Can you work these out from the model? Positions are in its coordinate system, mm. A direction names the side the tool comes from. Give positions to 0.01 mm unless a question says otherwise; leave off trailing zeros. Order: outer loops, then holes, each group sorted by start corner. A loop starts at its lowest first (then second) coordinate and runs counter-clockwise, first axis right, second up. Notation, with made-up numbers: M -31.5,53 L -7.5,53 A23 ccw -7.5,91 Z; hole C 15.5,0 d11. An arc over 180 degrees is marked long. One line per question, with ' | ' between items. Start each with the question number.
1) Thinking about a two-plate mould opening in X: for faces 6 (the flat face through (-5.83, 4.93, -73.97)), 7 (the flat face through (1.75, 5, 7)), 8 (the flat face through (-19.32, 4.96, -84.28)), which applies, +X half, -X half, draft (parallel to the pull), parting line (faces both ways), or undercut?
2) If we section it at A-A, the plane y = 3.25: Please give me the cut outline in (x, z), plus the area to 3 significant figures.
3) Please list where these lines run through material, in increasing order: line 1 along X through (y, z) = (2.25, -53.5); line 2 along X through (y, z) = (2.25, 7.5); line 3 along X through (y, z) = (5, -78). Write a range as [from, to].
4) If we section it at D-D, the plane x = -25.5: Please give me the cut outline in (y, z), plus the area to 3 significant figures.
5) If we section it at B-B, the plane x = -17: Please give me the cut outline in (y, z), plus the area to 3 significant figures.
6) If we section it at C-C, the plane z = 2: Please give me the cut outline in (x, y), plus the area to 4 significant figures.
7) For faces 1 (the flat face through (8.25, 5, 7)), 2 (the flat face through (-23.21, 5.04, -80.39)), 3 (the flat face through (0, 5, -27)), 4 (the flat face through (5, 1.75, 7)), 5 (the flat face through (5, 8.25, 7)), which set-ups out of +Z, -Z, +X, -X, +Y, -Y let a thin tool reach every point of the face, with its end or its side?
8) I'm going to push flat-ended pins straight in: pin 1 Ø3 at (x, z) = (4, 9) entering from +Y; pin 2 Ø1.5 at (x, y) = (0.5, 2) entering from -Z; pin 3 Ø7 at (x, z) = (4.5, 8) entering from -Y. Where does each tip first touch, or does it pass through?
Autodesk Inventor part; units mm, degrees
ref_plane "YZ Plane" through (0, 0, 0) normal (1, 0, 0) x (0, 1, 0)
ref_plane "XZ Plane" through (0, 0, 0) normal (0, 1, 0) x (-1, 0, 0)
ref_plane "XY Plane" through (0, 0, 0) normal (0, 0, 1) x (1, 0, 0)
sketch "Sketch1" plane through (0, 0, 0) normal (0, 1, 0) x (-1, 0, 0)
  line L0 (0, 0) -> (-10, 0)
  line L1 (-10, 0) -> (-10, -54)
  line L2 (0, -54) -> (0, 0)
  line L3 (0, -54) -> (28.2843, -82.2843)
  line L4 (0, -54) -> (40, -54) construction
  line L5 (28.2843, -82.2843) -> (21.2132, -89.3553)
  line L6 (21.2132, -89.3553) -> (-10, -58.1421)
  line L7 (-10, -58.1421) -> (-10, -54)
extrude "Extrusion1" add sketch "Sketch1" along normal blind 10
sketch "Sketch2" plane through (0, 0, 0) normal (0, 0, 1) x (1, 0, 0)
  line L0 (1.75, 1.75) -> (8.25, 1.75)
  line L1 (8.25, 1.75) -> (8.25, 8.25)
  line L2 (8.25, 8.25) -> (1.75, 8.25)
  line L3 (1.75, 8.25) -> (1.75, 1.75)
  point P0 (0, 0)
extrude "Extrusion2" add sketch "Sketch2" along normal blind 15
sketch "Sketch3" plane through (-28.2843, 0, -82.2843) normal (-0.7071, 0, -0.7071) x (-0.7071, 0, 0.7071)
  line L0 (-2.25, 2.25) -> (-7.75, 2.25)
  line L1 (-7.75, 2.25) -> (-7.75, 7.75)
  line L2 (-7.75, 7.75) -> (-2.25, 7.75)
  line L3 (-2.25, 7.75) -> (-2.25, 2.25)
  point P0 (38.1838, 0)
extrude "Extrusion3" cut sketch "Sketch3" against normal blind 10
properties part number "Stalk_v2"
Results found:
1) face 6: +X half | face 7: -X half | face 8: undercut
2) outline: M -28.28,-82.28 L -26.69,-83.88 L -19.62,-76.8 L -15.73,-80.69 L -22.8,-87.76 L -21.21,-89.36 L 10,-58.14 L 10,0 L 8.25,0 L 8.25,15 L 1.75,15 L 1.75,0 L 0,0 L 0,-54 Z | area: 1,020 mm²
3) line 1: x = [0, 10] | line 2: x = [1.75, 8.25] | line 3: x = [-24, -20.82], [-18.42, -9.86]
4) outline: M 0,-85.07 L 2.25,-85.07 L 2.25,-82.68 L 7.75,-82.68 L 7.75,-85.07 L 10,-85.07 L 10,-79.5 L 0,-79.5 Z | area: 42.6 mm²
5) outline: M 0,-85.14 L 10,-85.14 L 10,-71 L 0,-71 Z; hole M 2.25,-81.96 L 7.75,-81.96 L 7.75,-79.42 L 2.25,-79.42 Z | area: 127 mm²
6) outline: M 1.75,1.75 L 8.25,1.75 L 8.25,8.25 L 1.75,8.25 Z | area: 42.25 mm²
7) face 1: +Z, +X, +Y, -Y | face 2: none | face 3: +Z, -X, +Y, -Y | face 4: +Z, +X, -X, -Y | face 5: +Z, +X, -X, +Y
8) pin 1: stops at y = 8.25 | pin 2: stops at z = -68.39 | pin 3: stops at y = 1.75
